```python
from build123d import *

# Parameters (mm, degrees)
F0_W     = 7.31414
F0_H     = 3.485261
F1_DEPTH = 25.4
F3_D     = 2.8956
F5_D     = 2.8956


with BuildPart() as f1:
    # F0 (on Front) → F1 (new body)
    with BuildSketch(Plane.XZ):
        with Locations((-27.067565, 16.338196)):
            Rectangle(F0_W, F0_H)
    extrude(amount=F1_DEPTH)

    # F3 (through all)
    with Locations(Plane.XZ.offset(25.4)):
        with Locations((-29.874383, 16.361794)):
            Hole(F3_D / 2)

    # F5 (through all)
    with Locations(Plane.XZ.offset(25.4)):
        with Locations((-24.294116, 16.361794)):
            Hole(F5_D / 2)


solid = f1.part
```
Input: part model. Units: mm. Frame: model coordinates. Give positions to 0.01 mm unless a question says otherwise; leave off trailing zeros. Order: outer loops, then holes, each group sorted by start corner. A loop starts at its lowest first (then second) coordinate and runs counter-clockwise, first axis right, second up. Notation, with made-up numbers: M -38,75 L 8,75 A14 ccw 8,82 Z; hole C 83.25,-10.5 d11. An arc over 180 degrees is marked long. Return JSON: item names as keys, results as strings.
1) Section query D-D on z = 16.9. Output: boundary loops of the cut face in (x, y), and give its area (3 significant figures).
Taken from the geometry:
{"outline": "M -28.53,-25.4 L -25.64,-25.4 L -25.64,0 L -28.53,0 Z", "area": "73.5 mm2"}
2) Mould query, pull axis Z, two halves, no side actions, for faces 1 (the face through (-25.74, -12.52, 16.32)), 2 (the face through (-27, -13, 18.081)), 3 (the face through (-27, 0, 16)). Classes: released by +Z, released by -Z, zero draft, split by the parting line, or undercut.
Taken from the geometry:
{"face 1": "undercut", "face 2": "released by +Z", "face 3": "zero draft"}
3) Line query: L1, parallel to X at y = -19, z = 16.25; L2, parallel to Z at x = -23.75, y = -2.5; L3, parallel to Z at x = -24, y = -4. Output: solid intervals per line, ascending. Write a range as [from, to].
Taken from the geometry:
{"L1": "x = [-28.43, -25.74]", "L2": "z = [14.6, 15.02], [17.7, 18.08]", "L3": "z = [14.6, 14.94], [17.78, 18.08]"}
4) Contact query for a flat-ended pin moving along its axis: pin 1 (1.5 mm diameter, centred on y = -6.5, z = 17, fed in from +X). Output: stop coordinate, or through.
Taken from the geometry:
{"pin 1": "stops at x = -23.41"}
5) Section query C-C on x = -23.75. Output: boundary loops of the cut face in (y, z), and give its area (3 significant figures).
Taken from the geometry:
{"outline": "M -25.4,14.6 L 0,14.6 L 0,15.02 L -25.4,15.02 Z; M -25.4,17.7 L 0,17.7 L 0,18.08 L -25.4,18.08 Z", "area": "20.4 mm2"}
6) Section query A-A on x = -29.25. Output: boundary loops of the cut face in (y, z), and give its area (3 significant figures).
Taken from the geometry:
{"outline": "M -25.4,14.6 L 0,14.6 L 0,15.06 L -25.4,15.06 Z; M -25.4,17.67 L 0,17.67 L 0,18.08 L -25.4,18.08 Z", "area": "22.2 mm2"}
7) Section query B-B on y = -21.25. Output: boundary loops of the cut face in (x, z), and give its area (3 significant figures).
Taken from the geometry:
{"outline": "M -30.72,14.6 L -23.41,14.6 L -23.41,15.21 A1.45 cw long -23.41,17.51 L -23.41,18.08 L -30.72,18.08 L -30.72,17.53 A1.45 cw long -30.72,15.19 Z", "area": "14.2 mm2"}
